For this review, take the finished solid that the model builds, in its own axes (mm). Face numbers are marked on the shaded views. A direction names the side the tool comes from. Give positions to 0.01 mm unless a question says otherwise; leave off trailing zeros. Order: outer loops, then holes, each group sorted by start corner. A loop starts at its lowest first (then second) coordinate and runs counter-clockwise, first axis right, second up. Notation, with made-up numbers: (86.5, -19) - (138.5, -19) arc R10 ccw to (138.5, -2) - close; hole circle Ø4 at (4.5, -33). An arc over 180 degrees is marked (long way). One line per item, written item: value.
```python
from build123d import *

# Parameters (mm, degrees)
F0_W     = 136.94
F0_H     = 84.65
F1_DEPTH = 25
F2_W     = 108.94
F2_H     = 71.65
F2_H_2   = 2.5
F3_DEPTH = 22
F4_W     = 22
F4_H     = 80.65
F5_DEPTH = 22
F6_W     = 108.94
F6_H     = 2
F7_DEPTH = 20


with BuildPart() as f1:
    # F0 (on Top) → F1 (new body)
    with BuildSketch(Plane.XY):
        with Locations((68.47, 42.325)):
            Rectangle(F0_W, F0_H)
    extrude(amount=F1_DEPTH)

    # F2 (on face) → F3 (cut)
    with BuildSketch(Plane.XY.offset(25)):
        with Locations((56.47, 42.325)):
            Rectangle(F2_W, F2_H)
        with Locations((56.47, 3.25)):
            Rectangle(F2_W, F2_H_2)
        with Locations((56.47, 81.4)):
            Rectangle(F2_W, F2_H_2)
    extrude(amount=-F3_DEPTH, mode=Mode.SUBTRACT)

    # F4 (on face) → F5 (cut)
    with BuildSketch(Plane.XY.offset(25)):
        with Locations((123.94, 42.325)):
            Rectangle(F4_W, F4_H)
    extrude(amount=-F5_DEPTH, mode=Mode.SUBTRACT)

    # F6 (on face) → F7 (cut)
    with BuildSketch(Plane.XY.offset(25)):
        with Locations((56.47, 79.15)):
            Rectangle(F6_W, F6_H)
        with Locations((56.47, 5.5)):
            Rectangle(F6_W, F6_H)
    extrude(amount=-F7_DEPTH, mode=Mode.SUBTRACT)


solid = f1.part
```
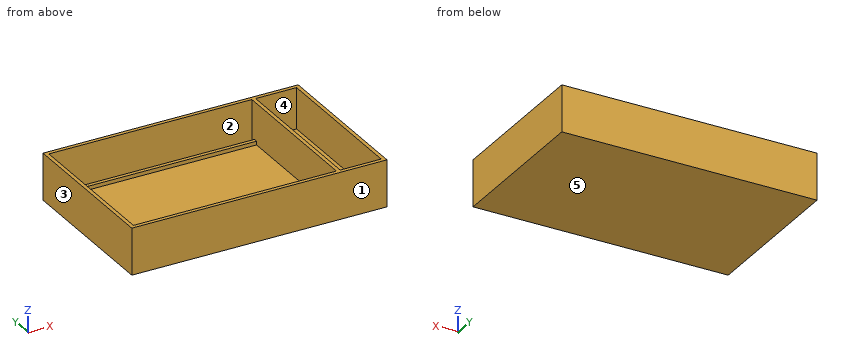
(1) Draft analysis for pull direction X (two halves, no side actions). For the marked faces 1, 2 and 3, state which applies: pulls with the +X half, pulls with the -X half, needs draft (parallel to the pull), parting line crosses it, or undercut.
Answers below:
face 1: needs draft
face 2: undercut
face 3: pulls with the -X half
(2) Take a section at C-C (y = 43). Write out the cut boundary in (x, z), then the cut area to 3 significant figures.
Answers below:
outline: (0, 0) - (136.94, 0) - (136.94, 25) - (134.94, 25) - (134.94, 3) - (112.94, 3) - (112.94, 25) - (110.94, 25) - (110.94, 3) - (2, 3) - (2, 25) - (0, 25) - close
area: 543 mm^2
(3) Take a section at D-D (x = 68). Write out the cut boundary in (y, z), then the cut area to 3 significant figures.
Answers below:
outline: (0, 0) - (84.65, 0) - (84.65, 25) - (82.65, 25) - (82.65, 3) - (80.15, 3) - (80.15, 5) - (78.15, 5) - (78.15, 3) - (6.5, 3) - (6.5, 5) - (4.5, 5) - (4.5, 3) - (2, 3) - (2, 25) - (0, 25) - close
area: 350 mm^2
(4) Take a section at B-B (x = 128.5). Write out the cut boundary in (y, z).
Answers below:
outline: (0, 0) - (84.65, 0) - (84.65, 25) - (82.65, 25) - (82.65, 3) - (2, 3) - (2, 25) - (0, 25) - close
(5) Wall thickness on line 1 (Y direction, x = 97, z = 3.25); line 2 (X direction, y = 22.5, z = 7.5); line 3 (Y direction, x = 24, z = 22.75): over which ranges is each line inside the solid? List them lowest first. Write a range as from..to.
Answers below:
line 1: y = 0..2, 4.5..6.5, 78.15..80.15, 82.65..84.65
line 2: x = 0..2, 110.94..112.94, 134.94..136.94
line 3: y = 0..2, 82.65..84.65
(6) Machinability: for the marked faces 4 and 5, which of the approach directions +Z, -Z, +X, -X, +Y, -Y give a long, thin tool a straight path to every point of the face, cutting with its end or side? Answer none if there is none.
Answers below:
face 4: +Z
face 5: -Z, +X, -X, +Y, -Y
(7) For P1, Ø2, axis at x = 58, y = 81.5, coming from the +Z side; P2, Ø1.6, axis at x = 44, y = 79.5, coming from the +Z side, all flat-tipped, find the tip position at first contact; note any pin that passes through.
Answers below:
P1: stops at z = 3
P2: stops at z = 5
(8) Take a section at A-A (z = 16.5). Write out the cut boundary in (x, y), then the cut area to 3 significant figures.
Answers below:
outline: (0, 0) - (136.94, 0) - (136.94, 84.65) - (0, 84.65) - close; hole (2, 2) - (110.94, 2) - (110.94, 82.65) - (2, 82.65) - close; hole (112.94, 2) - (134.94, 2) - (134.94, 82.65) - (112.94, 82.65) - close
area: 1,030 mm^2
